Check sheet for the drawn part. Datum: minimum x, y, z corner. Units: mm. A direction names the side the tool comes from. Coordinates: 2 decimals unless noted, no trailing zeros. Order: outer loops, then holes, each group sorted by start corner. A loop starts at its lowest first (then second) coordinate and runs counter-clockwise, first axis right, second up. Notation, with made-up numbers: (85, -12) - (123, -12) arc R13 ccw to (123, -3) - close; hole circle Ø9 at (19, -27). An arc over 180 degrees is marked (long way). Answer as CSV lines item,"result". Start each with the question number.
1. Section check C-C (x = 5.75). Record the cut outline in (y, z), and give its area (3 significant figures).
2. Section check A-A (z = 40). Record the cut outline in (x, y).
3. Go/stop test with flat-tipped pins: pin 1 (12 mm diameter, centred on x = 7.5, y = 13.5, fed in from +Z); pin 2 (2 mm diameter, centred on x = 17, z = 35.5, fed in from -Y); pin 3 (5 mm diameter, centred on x = 4.5, z = 44.5, fed in from +Y); pin 4 (6.5 mm diameter, centred on y = 30, z = 24, fed in from -X). Record where each tip stops, or that it passes through.
4. Set-up check for the marked faces 1, 2 and 3: record each of +Z, -Z, +X, -X, +Y, -Y from which the full face is reachable in a straight line by a thin tool's end or side.
5. Section check B-B (y = 30). Record the cut outline in (x, z).
6. Mould release check, pull along Y, two halves, no side actions. Record for the marked faces 4, 5, 6 and 7: pulls with the +Y half, pulls with the -Y half, needs draft (parallel to the pull), parting line crosses it, or undercut.
7. Material ranges on L1, parallel to Z at x = 7.25, y = 30; L2, parallel to Z at x = 17.5, y = 28.5; L3, parallel to Z at x = 12.5, y = 11, recorded low to high. Write a range as [from, to].
8. Section check D-D (y = 16). Record the cut outline in (x, z), and give its area (3 significant figures).
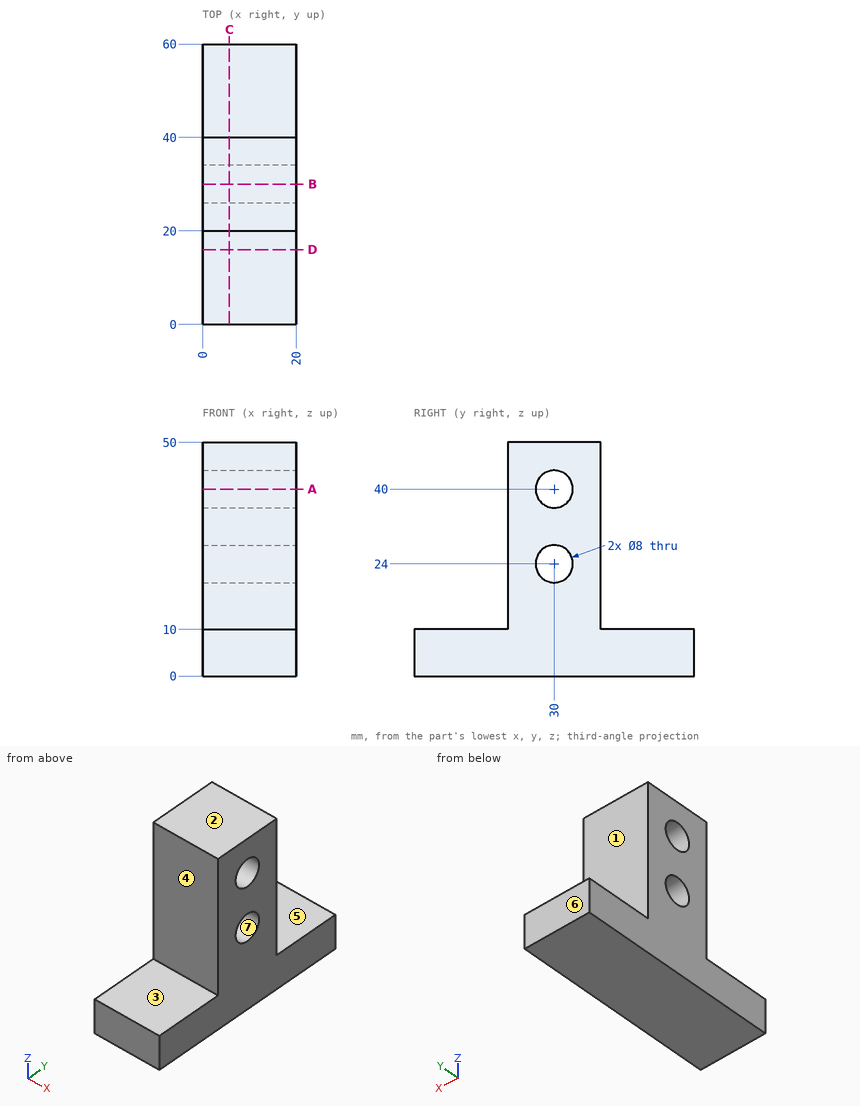
Evaluation:
1,outline,"(0, 0) - (60, 0) - (60, 10) - (40, 10) - (40, 50) - (20, 50) - (20, 10) - (0, 10) - close; hole circle Ø8 at (30, 24); hole circle Ø8 at (30, 40)"
1,area,"1,300 mm²"
2,outline,"(0, 20) - (20, 20) - (20, 26) - (0, 26) - close; (0, 34) - (20, 34) - (20, 40) - (0, 40) - close"
3,pin 1,"stops at z = 10"
3,pin 2,"stops at y = 20"
3,pin 3,"stops at y = 40"
3,pin 4,"passes through"
4,face 1,"+Z, +X, -X, +Y"
4,face 2,"+Z, +X, -X, +Y, -Y"
4,face 3,"+Z, +X, -X, -Y"
5,outline,"(0, 0) - (20, 0) - (20, 20) - (0, 20) - close; (0, 28) - (20, 28) - (20, 36) - (0, 36) - close; (0, 44) - (20, 44) - (20, 50) - (0, 50) - close"
6,face 4,"pulls with the -Y half"
6,face 5,"needs draft"
6,face 6,"pulls with the +Y half"
6,face 7,"undercut"
7,L1,"z = [0, 20], [28, 36], [44, 50]"
7,L2,"z = [0, 20.29], [27.71, 36.29], [43.71, 50]"
7,L3,"z = [0, 10]"
8,outline,"(0, 0) - (20, 0) - (20, 10) - (0, 10) - close"
8,area,"200 mm²"
